Work out the finished part from the listing and answer in its coordinate system (mm). A direction names the side the tool comes from. Coordinates: 2 decimals unless noted, no trailing zeros. Order: outer loops, then holes, each group sorted by start corner. A loop starts at its lowest first (then second) coordinate and runs counter-clockwise, first axis right, second up. Notation, with made-up numbers: (41, 34) -> (71, 34) arc R16 cw to (71, 39) -> close; hole circle Ø11 at (-19, -25). An arc over 180 degrees is marked (long way). Answer as CSV lines item,"result". Start each with the question number.
Item 1: Each of these flat-tipped pins is pushed along its axis until it touches: pin 1 Ø1.5 at (y, z) = (79.5, -18.5) entering from -X; pin 2 Ø19 at (y, z) = (40, -20) entering from +X; pin 3 Ø7 at (x, z) = (10, -23) entering from +Y; pin 4 Ø6 at (y, z) = (40, -20.5) entering from -X. Where does it stop, or does it pass through?
Item 2: Section C-C (z = -12) is taken. Write down the section's boundary in (x, y).
Item 3: Section A-A (y = 24.5) is taken. Count the separate pieces of the cut face and the enclosed holes in it, then the cut area to 3 significant figures.
Item 4: Section D-D (y = 102.5) is taken. Write down the section's boundary in (x, z), then the cut area to 3 significant figures.
Item 5: For a pull along X with two mould halves and no side action, classify faces 5 (the face through (84.708, 0.753, -36.302)), 6 (the face through (97.46, 36.35, -24.76)), 7 (the face through (49.441, -15.645, -36.198)) as pulls with the +X half, pulls with the -X half, needs draft (parallel to the pull), parting line crosses it, or undercut.
Item 6: Straight lines are drawn through the part: L1, parallel to Y at x = 2.8, z = -4.5; L2, parallel to Y at x = 95.05, z = -5.75; L3, parallel to X at y = 61, z = -36. For each, find the intervals that lie inside material, in ascending order.
Item 7: Which of the six approach directions +Z, -Z, +X, -X, +Y, -Y give full straight-line access (tool end or side, diameter ignored) to faces 1 (the face through (78.51, 87.14, -36.2)), 2 (the face through (9, 65, -5)), 3 (the face through (13.1, 15.86, -34.93)), 4 (the face through (12, 0, -20))?
```python
from build123d import *

# Parameters (mm, degrees)
SKETCH1_R               = 4
BOSS_EXTRUDE1_DEPTH     = 40
CUT_EXTRUDE1_DEPTH      = 160.033809299
CUT_EXTRUDE1_DEPTH_BACK = 160.033809299
SKETCH2_W               = 100
SKETCH2_H               = 25
SKETCH3_W               = 25
SKETCH3_H               = 25
BOSS_EXTRUDE2_DEPTH     = 10
SKETCH4_R               = 6
CUT_EXTRUDE2_DEPTH      = 100
FILLET1_R               = 5
FILLET2_R               = 3
SKETCH5_R               = 1.75
CUT_EXTRUDE3_DEPTH      = 10
SKETCH7_W               = 10
SKETCH7_H               = 50
CUT_EXTRUDE4_DEPTH      = 10
FILLET3_R               = 3
FILLET3_OF_MIRROR1_R    = 3


with BuildPart() as part:
    # Sketch1 → Boss-Extrude1 (new body)
    with BuildSketch(Plane.XY):
        with BuildLine():
            Line((25, 0), (73.308886978, -30.922345302))
            ThreePointArc((73.308886978, -30.922345302), (80.218691228, -32.384006119), (86.370944241, -28.915342115))
            Line((86.370944241, -28.915342115), (102.720944241, -9.365342115))
            ThreePointArc((102.720944241, -9.365342115), (104.608588105, -5.888263678), (105, -1.951250782))
            Line((105, -1.951250782), (105, 0))
            Line((105, 0), (105, 80))
            Line((105, 80), (105, 81.951250782))
            ThreePointArc((105, 81.951250782), (104.608588105, 85.888263678), (102.720944241, 89.365342115))
            Line((102.720944241, 89.365342115), (86.370944241, 108.915342115))
            ThreePointArc((86.370944241, 108.915342115), (80.218691228, 112.384006119), (73.308886978, 110.922345302))
            Line((73.308886978, 110.922345302), (25, 80))
            Line((25, 80), (0, 80))
            Line((0, 80), (0, 0))
            Line((0, 0), (25, 0))
        make_face()
        with Locations((78.7, -22.5)):
            Circle(SKETCH1_R, mode=Mode.SUBTRACT)
        with Locations((95.05, -2.95)):
            Circle(SKETCH1_R, mode=Mode.SUBTRACT)
        with Locations(Location((78.7, 102.5, 0), (0, 0, 180))):
            Circle(SKETCH1_R, mode=Mode.SUBTRACT)
        with Locations(Location((95.05, 82.95, 0), (0, 0, 180))):
            Circle(SKETCH1_R, mode=Mode.SUBTRACT)
        Polygon((30.852797713, 71.873177413), (30.852797713, 8.126822587), (70.209148437, -17.065036365), (85, 0.620660764), (85, 79.379339236), (70.209148437, 97.065036365), align=None, mode=Mode.SUBTRACT)
    extrude(amount=-BOSS_EXTRUDE1_DEPTH)

    # Sketch2 → Cut-Extrude1 (cut, two sides: drawn at the far end of the back side and taken through both)
    with BuildSketch(Plane(origin=(0, 0, 0), x_dir=(1, 0, 0), z_dir=(0, 1, 0)).offset(-CUT_EXTRUDE1_DEPTH_BACK)):
        with Locations((70, 20)):
            Rectangle(SKETCH2_W, SKETCH2_H)
    extrude(amount=CUT_EXTRUDE1_DEPTH + CUT_EXTRUDE1_DEPTH_BACK, mode=Mode.SUBTRACT)

    # Sketch3 → Boss-Extrude2 (add)
    with BuildSketch(Plane(origin=(105, 0, 0), x_dir=(0, 0, -1), z_dir=(1, 0, 0))):
        with Locations((20, 40)):
            Rectangle(SKETCH3_W, SKETCH3_H)
    extrude(amount=-BOSS_EXTRUDE2_DEPTH)

    # Sketch4 → Cut-Extrude2 (cut)
    with BuildSketch(Plane.ZY):
        with Locations((-20, 40)):
            Circle(SKETCH4_R)
    extrude(amount=-CUT_EXTRUDE2_DEPTH, mode=Mode.SUBTRACT)

    # Fillet1
    fillet1_edges = [part.edges().sort_by_distance(p)[0] for p in [
        (25, 80, -3.75),
        (25, 80, -36.25),
        (25, 0, -36.25),
        (85, 79.379339236, -36.25),
        (85, 0.620660764, -36.25),
        (70.209148437, -17.065036365, -36.25),
        (30.852797713, 8.126822587, -36.25),
        (30.852797713, 71.873177413, -36.25),
        (70.209148437, 97.065036365, -36.25),
        (70.209148437, 97.065036365, -3.75),
        (85, 79.379339236, -3.75),
        (30.852797713, 71.873177413, -3.75),
        (30.852797713, 8.126822587, -3.75),
        (70.209148437, -17.065036365, -3.75),
        (85, 0.620660764, -3.75),
        (25, 0, -3.75),
    ]]
    fillet(fillet1_edges, radius=FILLET1_R)

    # Fillet2
    fillet2_edges = [part.edges().sort_by_distance(p)[0] for p in [
        (20, 40, -32.5),
        (20, 40, -7.5),
        (95, 40, -32.5),
        (95, 40, -7.5),
    ]]
    fillet(fillet2_edges, radius=FILLET2_R)

    # Sketch5 → Cut-Extrude3 (cut)
    with BuildSketch(Plane.ZY):
        with Locations((-35.5, 55.5)):
            Circle(SKETCH5_R)
        with Locations((-4.5, 55.5)):
            Circle(SKETCH5_R)
        with Locations((-35.5, 24.5)):
            Circle(SKETCH5_R)
        with Locations((-4.5, 24.5)):
            Circle(SKETCH5_R)
    extrude(amount=-CUT_EXTRUDE3_DEPTH, mode=Mode.SUBTRACT)

    # Sketch7 → Cut-Extrude4 (cut)
    with BuildSketch(Plane.XY):
        with Locations((9, 40)):
            Rectangle(SKETCH7_W, SKETCH7_H)
    cut_extrude4 = extrude(amount=-CUT_EXTRUDE4_DEPTH, mode=Mode.SUBTRACT)

    # Fillet3
    fillet3_edges = [part.edges().sort_by_distance(p)[0] for p in [
        (4, 15, -5),
        (4, 65, -5),
        (14, 65, -5),
        (14, 15, -5),
    ]]
    fillet(fillet3_edges, radius=FILLET3_R)

    # Mirror1: Cut-Extrude4 across plane
    add(cut_extrude4.mirror(Plane.XY.offset(-20)), mode=Mode.SUBTRACT)

    # Fillet3 of Mirror1
    fillet3_of_mirror1_edges = [part.edges().sort_by_distance(p)[0] for p in [
        (4, 15, -35),
        (4, 65, -35),
        (14, 65, -35),
        (14, 15, -35),
    ]]
    fillet(fillet3_of_mirror1_edges, radius=FILLET3_OF_MIRROR1_R)


solid = part.part
```
Checked values:
1,pin 1,"stops at x = 0"
1,pin 2,"stops at x = 105"
1,pin 3,"stops at y = 80"
1,pin 4,"stops at x = 100"
2,outline,"(0, 0) -> (20, 0) -> (20, 80) -> (0, 80) -> close; (95, 27.5) -> (105, 27.5) -> (105, 52.5) -> (95, 52.5) -> close"
3,separate pieces,"5"
3,enclosed holes,"0"
3,area,"1,040 mm^2"
4,outline,"(60.15, -40) -> (74.7, -40) -> (74.7, -32.5) -> (60.15, -32.5) -> close; (60.15, -7.5) -> (74.7, -7.5) -> (74.7, 0) -> (60.15, 0) -> close; (82.7, -40) -> (91.74, -40) -> (91.74, -32.5) -> (82.7, -32.5) -> close; (82.7, -7.5) -> (91.74, -7.5) -> (91.74, 0) -> (82.7, 0) -> close"
4,area,"354 mm^2"
5,face 5,"undercut"
5,face 6,"needs draft"
5,face 7,"pulls with the -X half"
6,L1,"y = 0 to 22.75, 26.25 to 53.75, 57.25 to 80"
6,L2,"y = -18.54 to -6.95, 1.05 to 78.95, 86.95 to 98.54"
6,L3,"x = 0 to 4, 14 to 30.85, 85 to 105"
7,face 1,"+Z, -Z"
7,face 2,"+Z"
7,face 3,"-Z"
7,face 4,"+Z, -Z, -X, -Y"
